from build123d import *

# Parameters (mm, degrees)
ESQUISSE1_W        = 3.5
ESQUISSE1_H        = 5
ESQUISSE1_W_2      = 5
ESQUISSE1_H_2      = 3.5
ESQUISSE1_W_3      = 4
BOSS_EXTRU_1_DEPTH = 380


with BuildPart() as part:
    # Esquisse1 → Boss.-Extru.1 (new body)
    with BuildSketch(Plane.XY):
        Polygon((7.5, 16), (7.5, 20), (0, 20), (4, 16), align=None)
        Polygon((4, 16), (0, 20), (0, 12.5), (4, 12.5), align=None)
        Polygon((4, 7.5), (0, 7.5), (0, 0), (4, 4), align=None)
        Polygon((0, 0), (7.5, 0), (7.5, 4), (4, 4), align=None)
        Polygon((4, 4), (7.5, 7.5), (4, 7.5), align=None)
        Polygon((7.5, 4), (7.5, 7.5), (4, 4), align=None)
        Polygon((4, 12.5), (7.5, 12.5), (4, 16), align=None)
        Polygon((7.5, 12.5), (7.5, 16), (4, 16), align=None)
        with Locations((5.75, 10)):
            Rectangle(ESQUISSE1_W, ESQUISSE1_H)
        Polygon((7.5, 7.5), (10, 10), (7.5, 12.5), align=None)
        Polygon((10, 10), (12.5, 12.5), (7.5, 12.5), align=None)
        Polygon((12.5, 7.5), (12.5, 12.5), (10, 10), align=None)
        Polygon((12.5, 7.5), (10, 10), (7.5, 7.5), align=None)
        Polygon((16, 4), (12.5, 7.5), (12.5, 4), align=None)
        Polygon((16, 4), (16, 7.5), (12.5, 7.5), align=None)
        Polygon((20, 0), (20, 7.5), (16, 7.5), (16, 4), align=None)
        with Locations((10, 14.25)):
            Rectangle(ESQUISSE1_W_2, ESQUISSE1_H_2)
        with Locations((14.25, 10)):
            Rectangle(ESQUISSE1_W, ESQUISSE1_H)
        Polygon((12.5, 12.5), (16, 16), (12.5, 16), align=None)
        Polygon((16, 16), (20, 20), (12.5, 20), (12.5, 16), align=None)
        Polygon((16, 12.5), (16, 16), (12.5, 12.5), align=None)
        Polygon((20, 12.5), (20, 20), (16, 16), (16, 12.5), align=None)
        Polygon((12.5, 0), (20, 0), (16, 4), (12.5, 4), align=None)
        with Locations((10, 5.75)):
            Rectangle(ESQUISSE1_W_2, ESQUISSE1_H_2)
        with Locations((18, 10)):
            Rectangle(ESQUISSE1_W_3, ESQUISSE1_H)
        with Locations((22, 10)):
            Rectangle(ESQUISSE1_W_3, ESQUISSE1_H)
        Polygon((24, 16), (20, 20), (20, 12.5), (24, 12.5), align=None)
        Polygon((27.5, 20), (20, 20), (24, 16), (27.5, 16), align=None)
        Polygon((27.5, 12.5), (24, 16), (24, 12.5), align=None)
        Polygon((27.5, 16), (24, 16), (27.5, 12.5), align=None)
        with Locations((25.75, 10)):
            Rectangle(ESQUISSE1_W, ESQUISSE1_H)
        Polygon((27.5, 7.5), (24, 7.5), (24, 4), align=None)
        Polygon((24, 7.5), (20, 7.5), (20, 0), (24, 4), align=None)
        Polygon((24, 4), (20, 0), (27.5, 0), (27.5, 4), align=None)
        Polygon((27.5, 4), (27.5, 7.5), (24, 4), align=None)
        with Locations((30, 5.75)):
            Rectangle(ESQUISSE1_W_2, ESQUISSE1_H_2)
        Polygon((36, 4), (32.5, 7.5), (32.5, 4), align=None)
        Polygon((36, 7.5), (32.5, 7.5), (36, 4), align=None)
        Polygon((40, 0), (40, 7.5), (36, 7.5), (36, 4), align=None)
        Polygon((32.5, 4), (32.5, 0), (40, 0), (36, 4), align=None)
        with Locations((34.25, 10)):
            Rectangle(ESQUISSE1_W, ESQUISSE1_H)
        Polygon((32.5, 12.5), (30, 10), (32.5, 7.5), align=None)
        Polygon((32.5, 7.5), (30, 10), (27.5, 7.5), align=None)
        Polygon((30, 10), (27.5, 12.5), (27.5, 7.5), align=None)
        Polygon((32.5, 12.5), (27.5, 12.5), (30, 10), align=None)
        Polygon((36, 16), (32.5, 12.5), (36, 12.5), align=None)
        Polygon((36, 16), (32.5, 16), (32.5, 12.5), align=None)
        Polygon((40, 20), (32.5, 20), (32.5, 16), (36, 16), align=None)
        Polygon((40, 12.5), (40, 20), (36, 16), (36, 12.5), align=None)
        with Locations((30, 14.25)):
            Rectangle(ESQUISSE1_W_2, ESQUISSE1_H_2)
    extrude(amount=BOSS_EXTRU_1_DEPTH)


solid = part.part
Design review of the part built by this model. Coordinates are the model's own, in mm. Give positions to 0.01 mm unless a question says otherwise; leave off trailing zeros. Loops run counter-clockwise (first coordinate to the right, second up) from the corner with the lowest first, then second, coordinate; pieces in that order, holes last. Notation, with made-up numbers: M 75.5,79 L 115.5,79 A17 ccw 115.5,105 Z; hole C -8.75,8.25 d10. An arc over 180 degrees is marked long. Write item = value, one per line.
Q1. We need section A-A (z = 55.5). Give the boundary of the cut face in (x, y), plus the area to 3 significant figures.
Output values:
outline = M 0,0 L 7.5,0 L 7.5,4 L 12.5,4 L 12.5,0 L 27.5,0 L 27.5,4 L 32.5,4 L 32.5,0 L 40,0 L 40,7.5 L 36,7.5 L 36,12.5 L 40,12.5 L 40,20 L 32.5,20 L 32.5,16 L 27.5,16 L 27.5,20 L 12.5,20 L 12.5,16 L 7.5,16 L 7.5,20 L 0,20 L 0,12.5 L 4,12.5 L 4,7.5 L 0,7.5 Z
area = 680 mm^2
Q2. To check wall thickness, follow line 1 (X direction, y = 16.25, z = 133.5); line 2 (Y direction, x = 38, z = 238); line 3 (X direction, y = 10.5, z = 124). State the ranges of each line that lie inside material, in increasing order. Write a range as [from, to].
Output values:
line_1 = [0, 7.5], [12.5, 27.5], [32.5, 40]
line_2 = [0, 7.5], [12.5, 20]
line_3 = [4, 36]
Q3. Insertion check: pin 1 (2.5 mm diameter, centred on x = 29.5, z = 231.5, fed in from -Y). The pin has a flat end and moves straight along its axis. Give the tip position at first contact, or say it passes through.
Output values:
pin_1 = 4
